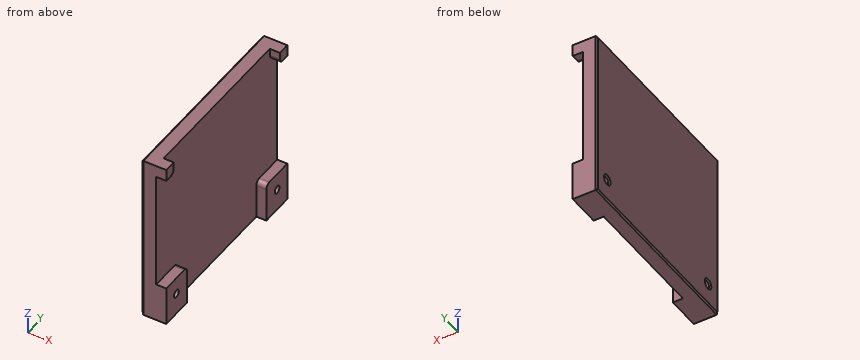
from build123d import *

# Parameters (mm, degrees)
SKETCH1_W           = 40.64
SKETCH1_H           = 35.56
BOSS_EXTRUDE1_DEPTH = 3
SKETCH3_W           = 7.0036
SKETCH3_H           = 8.1974
SKETCH3_W_2         = 2.5
SKETCH3_H_2         = 2.5
BOSS_EXTRUDE2_DEPTH = 2.1
SKETCH4_R           = 0.8
CUT_EXTRUDE2_DEPTH  = 28.47800575
FILLET1_R           = 1
CHAMFER1_SIZE       = 0.3


with BuildPart() as part:
    # Sketch1 → Boss-Extrude1 (new body)
    with BuildSketch(Plane.YZ):
        Rectangle(SKETCH1_W, SKETCH1_H)
    extrude(amount=BOSS_EXTRUDE1_DEPTH)

    # Sketch3 → Boss-Extrude2 (add)
    with BuildSketch(Plane.YZ.offset(3)):
        with Locations((-16.8182, -13.6813)):
            Rectangle(SKETCH3_W, SKETCH3_H)
        with Locations((16.8182, -13.6813)):
            Rectangle(SKETCH3_W, SKETCH3_H)
        with Locations((19.07, 16.53)):
            Rectangle(SKETCH3_W_2, SKETCH3_H_2)
        with Locations((-19.07, 16.53)):
            Rectangle(SKETCH3_W_2, SKETCH3_H_2)
    extrude(amount=BOSS_EXTRUDE2_DEPTH)

    # Sketch4 → Cut-Extrude2 (cut, through all)
    with BuildSketch(Plane.YZ.offset(5.1)):
        with Locations(Location((-16.9164, -13.1826, 0), (0, 0, 270))):
            Circle(SKETCH4_R)
        with Locations(Location((16.9164, -13.1826, 0), (0, 0, 270))):
            Circle(SKETCH4_R)
    extrude(amount=-CUT_EXTRUDE2_DEPTH, mode=Mode.SUBTRACT)

    # Fillet1
    fillet1_edges = [part.edges().sort_by_distance(p)[0] for p in [
        (4.05, -17.82, 15.28),
        (4.05, 17.82, 15.28),
        (4.05, 13.3164, -9.5826),
        (4.05, -13.3164, -9.5826),
    ]]
    fillet(fillet1_edges, radius=FILLET1_R)

    # Chamfer1
    chamfer1_edges = [part.edges().sort_by_distance(p)[0] for p in [
        (0, 0, -17.78),
        (0, -20.32, 0),
        (0, 0, 17.78),
        (0, -16.9164, -12.3826),
        (0, 20.32, 0),
        (0, 16.9164, -12.3826),
    ]]
    chamfer(chamfer1_edges, length=CHAMFER1_SIZE)


solid = part.part
The listing builds one solid part. Answer for the finished solid, in the listing's coordinates (mm). Round coordinates to 2 decimals unless told otherwise and drop trailing zeros. Order: outer loops, then holes, each group sorted by start corner. A loop starts at its lowest first (then second) coordinate and runs counter-clockwise, first axis right, second up. Notation, with made-up numbers: M -28,61.25 L 12,61.25 A12 ccw 12,84.25 Z; hole C 31.25,25.5 d3. An arc over 180 degrees is marked long. Answer in a Markdown table with one row per item. Add a question column.
1) The part is cut by section B-B on z = -15. Determine the outline of the cut face in (x, y).
2) The part is cut by section A-A on x = 4.05. Determine the outline of the cut face in (y, z), plus the area to 3 significant figures.
3) The part is cut by section C-C on y = -3. Determine the outline of the cut face in (x, z).
4) Flat-ended cylindrical pins translate along their axes: pin 1 Ø1.7 at (x, y) = (4.5, 17.5) entering from +Z; pin 2 Ø10.5 at (y, z) = (-5, -2) entering from +X. Find the tip coordinate at first contact, or state that the pin passes through.
5) Consider line 1 along Y through (x, z) = (4.2, -12); line 2 along X through (y, z) = (8, 12.5); line 3 along Y through (x, z) = (2.7, -12.5). Determine where each line is inside the solid, lowest interval first. Write a range as from..to.
6) The part is cut by section D-D on z = 3.5. Determine the outline of the cut face in (x, y), plus the area to 3 significant figures.
Findings below:
| question | item | result |
|---|---|---|
| 1 | outline | M 0,-20.02 L 0.3,-20.32 L 5.1,-20.32 L 5.1,-13.32 L 3,-13.32 L 3,13.32 L 5.1,13.32 L 5.1,20.32 L 0.3,20.32 L 0,20.02 Z |
| 2 | outline | M -20.32,-17.78 L -13.32,-17.78 L -13.32,-10.58 A1 ccw -14.32,-9.58 L -20.32,-9.58 Z; M -20.32,15.28 L -18.82,15.28 A1 ccw -17.82,16.28 L -17.82,17.78 L -20.32,17.78 Z; M 13.32,-17.78 L 20.32,-17.78 L 20.32,-9.58 L 14.32,-9.58 A1 ccw 13.32,-10.58 Z; M 17.82,16.28 A1 ccw 18.82,15.28 L 20.32,15.28 L 20.32,17.78 L 17.82,17.78 Z; hole C -16.92,-13.18 d1.6; hole C 16.92,-13.18 d1.6 |
| 2 | area | 122 mm² |
| 3 | outline | M 0,-17.48 L 0.3,-17.78 L 3,-17.78 L 3,17.78 L 0.3,17.78 L 0,17.48 Z |
| 4 | pin 1 | stops at z = 17.78 |
| 4 | pin 2 | stops at x = 3 |
| 5 | line 1 | y = -20.32..-13.32, 13.32..20.32 |
| 5 | line 2 | x = 0..3 |
| 5 | line 3 | y = -20.32..-17.33, -16.5..16.5, 17.33..20.32 |
| 6 | outline | M 0,-20.02 L 0.3,-20.32 L 3,-20.32 L 3,20.32 L 0.3,20.32 L 0,20.02 Z |
| 6 | area | 122 mm² |
